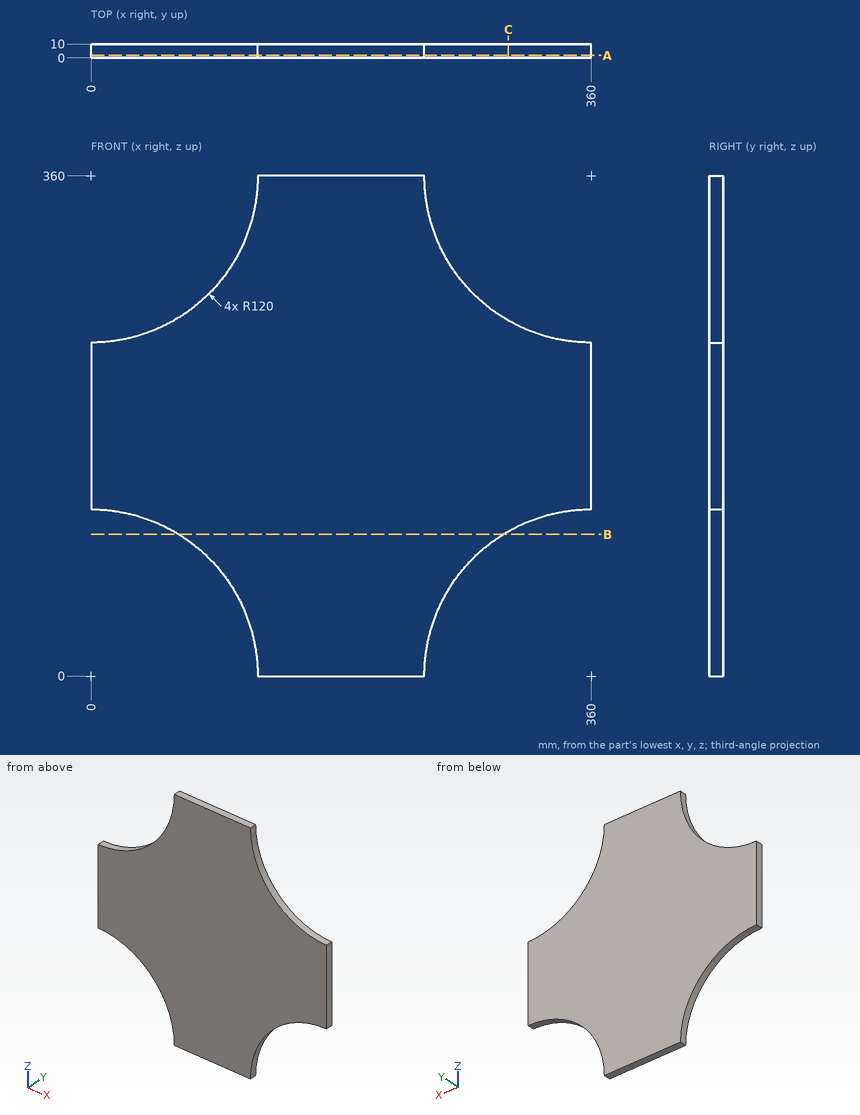
Part print with two shaded views. Sizes in mm from the minimum x, y, z corner. Round coordinates to 2 decimals unless told otherwise and drop trailing zeros. Order: outer loops, then holes, each group sorted by start corner. A loop starts at its lowest first (then second) coordinate and runs counter-clockwise, first axis right, second up. Notation, with made-up numbers: (11.25, 76.5) -> (22.25, 76.5) arc R22 cw to (22.25, 102.5) -> close; hole circle Ø2 at (77, 5). An arc over 180 degrees is marked (long way). One line per question, with ' | ' between items.
Q1. Slice it at B-B (z = 102). Write the cut outline in (x, y), then the cut area to 3 significant figures.
Completed:
outline: (63.21, 0) -> (296.79, 0) -> (296.79, 10) -> (63.21, 10) -> close | area: 2,340 mm^2
Q2. Probe probe 1 along X at (y, z) = (2, 70.5); probe 2 along X at (y, z) = (0.5, 44.5); probe 3 along Z at (x, y) = (65, 7.5). List the from-to ranges inside material, lowest first.
Completed:
probe 1: x = 97.11 to 262.89 | probe 2: x = 111.44 to 248.56 | probe 3: z = 100.87 to 259.13
Q3. Drop flat-ended pins along their axis: pin 1 (4 mm diameter, centred on x = 280, y = 3, fed in from +Z); pin 2 (1 mm diameter, centred on y = 9, z = 69.5, fed in from -X); pin 3 (1.5 mm diameter, centred on y = 5.5, z = 309.5, fed in from -X). Give the stop position or say it passes through.
Completed:
pin 1: stops at z = 272.39 | pin 2: stops at x = 97.47 | pin 3: stops at x = 108.51
Q4. Slice it at C-C (x = 300.5). Write the cut outline in (y, z).
Completed:
outline: (0, 104.21) -> (10, 104.21) -> (10, 255.79) -> (0, 255.79) -> close
Q5. Slice it at A-A (y = 1.75). Write the cut outline in (x, z).
Completed:
outline: (0, 120) arc R120 cw to (120, 0) -> (240, 0) arc R120 cw to (360, 120) -> (360, 240) arc R120 cw to (240, 360) -> (120, 360) arc R120 cw to (0, 240) -> close
